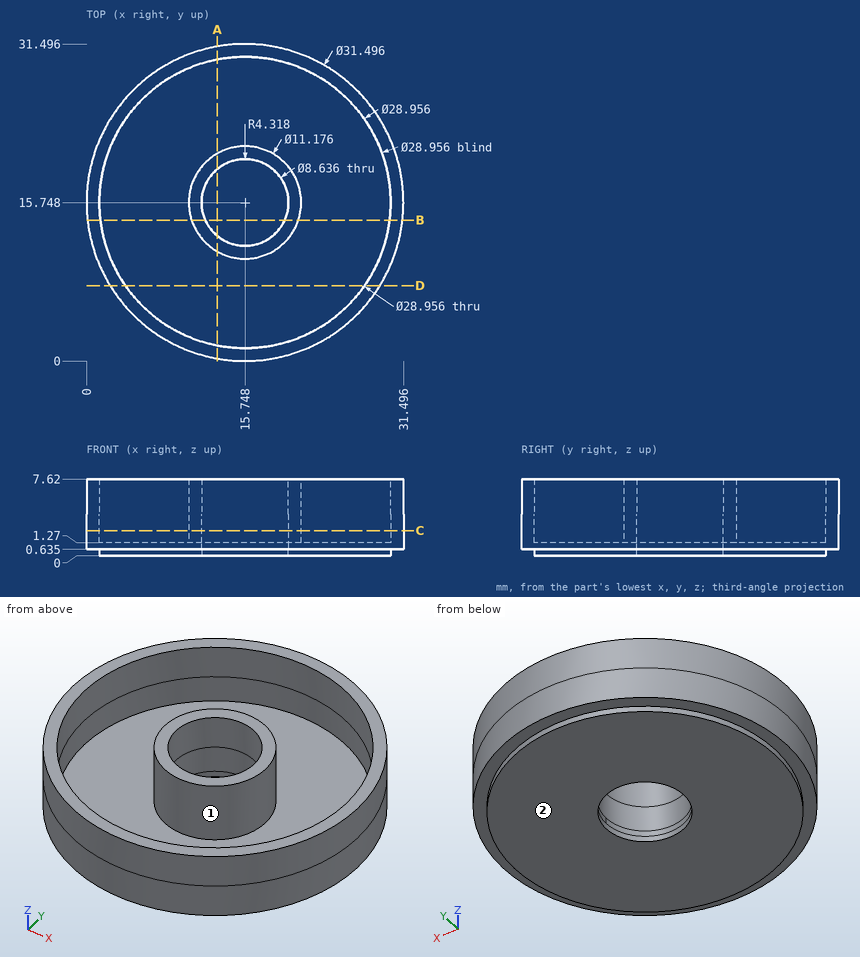
Job drawing, mm, ordinate dimensions from the low corner. One solid piece. A direction names the side the tool comes from. Coordinates: 2 decimals unless noted, no trailing zeros. Order: outer loops, then holes, each group sorted by start corner. A loop starts at its lowest first (then second) coordinate and runs counter-clockwise, first axis right, second up. Notation, with made-up numbers: (28, 51.25) -> (80, 51.25) arc R21 ccw to (80, 87.25) -> close; hole circle Ø8 at (-2, -2.5). An arc over 180 degrees is marked (long way). Return JSON: item names as keys, results as strings. Group by question number.
Item 1: Saw through at A-A on x = 13. Write the cut outline in (y, z) (3 decimals), then the cut area to 3 significant figures.
Item 2: Wall check: line 1 along Y through (x, z) = (16, 3.75); line 2 along X through (y, z) = (17.5, 6.25); line 3 along X through (y, z) = (18, 4.5). Give the ranges that are in metal, low to high. Write a range as [from, to].
Item 3: Saw through at C-C on z = 2.5. Write the cut outline in (x, y), then the cut area to 3 significant figures.
Item 4: Flat gauge pins, fed straight in: P1, Ø4, axis at x = 14.5, y = 28, coming from the +Z side; P2, Ø1, axis at x = 9, z = 6.5, coming from the +Y side; P3, Ø7, axis at x = 15.748, y = 15.748, coming from the +Z side; P4, Ø1, axis at x = 4, z = 2, coming from the +Y side. Where does each tip first touch, or does it go through?
Item 5: Tool access for the marked faces 1 and 2: list every direction of +Z, -Z, +X, -X, +Y, -Y with a clear straight run to the whole face (end or side of a thin tool).
Item 6: Saw through at B-B on y = 14. Write the cut outline in (x, z) (3 decimals), then the cut area to 3 significant figures.
Item 7: Saw through at D-D on y = 7.5. Write the cut outline in (x, z) (3 decimals).
Values found:
{
 "1": {"outline": "(0.242, 0.635) -> (1.533, 0.635) -> (1.533, 0) -> (12.417, 0) -> (12.417, 7.62) -> (10.882, 7.62) -> (10.882, 1.27) -> (1.533, 1.27) -> (1.533, 7.62) -> (0.242, 7.62) -> close; (19.079, 0) -> (29.963, 0) -> (29.963, 0.635) -> (31.254, 0.635) -> (31.254, 7.62) -> (29.963, 7.62) -> (29.963, 1.27) -> (20.614, 1.27) -> (20.614, 7.62) -> (19.079, 7.62) -> close", "area": "65.2 mm2"},
 "2": {"line 1": "y = [0, 1.27], [10.17, 11.44], [20.06, 21.33], [30.22, 31.49]", "line 2": "x = [0.1, 1.38], [10.44, 11.8], [19.69, 21.05], [30.12, 31.4]", "line 3": "x = [0.16, 1.45], [10.63, 12.06], [19.43, 20.86], [30.05, 31.33]"},
 "3": {"outline": "circle Ø31.5 at (15.75, 15.75); circle Ø11.18 at (15.75, 15.75); hole circle Ø28.96 at (15.75, 15.75); hole circle Ø8.64 at (15.75, 15.75)", "area": "160 mm2"},
 "4": {"P1": "stops at z = 1.27", "P2": "stops at y = 30.2", "P3": "passes through", "P4": "stops at y = 26.77"},
 "5": {"face 1": "+Z", "face 2": "-Z, +X, -X, +Y, -Y"},
 "6": {"outline": "(0.097, 0.635) -> (1.376, 0.635) -> (1.376, 0) -> (11.8, 0) -> (11.8, 7.62) -> (10.44, 7.62) -> (10.44, 1.27) -> (1.376, 1.27) -> (1.376, 7.62) -> (0.097, 7.62) -> close; (19.696, 0) -> (30.12, 0) -> (30.12, 0.635) -> (31.399, 0.635) -> (31.399, 7.62) -> (30.12, 7.62) -> (30.12, 1.27) -> (21.056, 1.27) -> (21.056, 7.62) -> (19.696, 7.62) -> close", "area": "61.6 mm2"},
 "7": {"outline": "(2.333, 0.635) -> (3.849, 0.635) -> (3.849, 0) -> (27.647, 0) -> (27.647, 0.635) -> (29.163, 0.635) -> (29.163, 7.62) -> (27.647, 7.62) -> (27.647, 1.27) -> (3.849, 1.27) -> (3.849, 7.62) -> (2.333, 7.62) -> close"}
}
